from build123d import *

# Parameters (mm, degrees)
SKETCH1_R               = 1.995
BOSS_EXTRUDE1_DEPTH     = 38
SKETCH2_W               = 4.5
SKETCH2_H               = 0.920377874
CUT_EXTRUDE1_DEPTH      = 2.995
CUT_EXTRUDE1_DEPTH_BACK = 2.995
CHAMFER1_SIZE           = 0.2


with BuildPart() as part:
    # Sketch1 → Boss-Extrude1 (new body)
    with BuildSketch(Plane.XY):
        Circle(SKETCH1_R)
    extrude(amount=BOSS_EXTRUDE1_DEPTH)

    # Sketch2 → Cut-Extrude1 (cut, two sides)
    with BuildSketch(Plane(origin=(0, 0, 0), x_dir=(0, 0, -1), z_dir=(1, 0, 0))) as cut_extrude1_sk:
        with Locations((-3.75, 2.160188937)):
            Rectangle(SKETCH2_W, SKETCH2_H)
        with Locations((-3.75, -2.160188937)):
            Rectangle(SKETCH2_W, SKETCH2_H)
    extrude(amount=CUT_EXTRUDE1_DEPTH, mode=Mode.SUBTRACT)
    extrude(cut_extrude1_sk.sketch, amount=-CUT_EXTRUDE1_DEPTH_BACK, mode=Mode.SUBTRACT)

    # Chamfer1
    chamfer1_edges = [part.edges().sort_by_distance(p)[0] for p in [
        (-1.995, 0, 0),
        (-1.995, 0, 38),
    ]]
    chamfer(chamfer1_edges, length=CHAMFER1_SIZE)


solid = part.part
Verification items for the finished model (mm, model axes). A direction names the side the tool comes from. Coordinates: 2 decimals unless noted, no trailing zeros. Order: outer loops, then holes, each group sorted by start corner. A loop starts at its lowest first (then second) coordinate and runs counter-clockwise, first axis right, second up. Notation, with made-up numbers: (69, 63.5) -> (115, 63.5) arc R19 cw to (115, 79.5) -> close; hole circle Ø8 at (-33, 2). An arc over 180 degrees is marked (long way). Put each result on its own line as item: value. Start each with the question number.
1. Cross-section at A-A, the plane x = 0. Record the boundary of the cut face in (y, z) (3 decimals), then the cut area to 3 significant figures.
2. Cross-section at B-B, the plane z = 15. Record the boundary of the cut face in (x, y) (3 decimals), then the cut area to 3 significant figures.
3. Go/stop test with flat-tipped pins: pin 1 Ø1 at (x, z) = (1, 27) entering from -Y; pin 2 Ø1.5 at (x, z) = (-1.5, 9) entering from -Y; pin 3 Ø0.6 at (x, z) = (0, 3) entering from +Y. Record where each tip stops, or that it passes through.
4. Material ranges on L1, parallel to Y at x = 0.1, z = 17.5; L2, parallel to X at y = -1.05, z = 22; L3, parallel to Y at x = 1.4, z = 7, recorded low to high. Write a range as [from, to].
5. Mould release check, pull along Z, two halves, no side actions. Record for faces 1 (the cylindrical face through (-0.26, 1.98, 18.74)), 2 (the flat face through (0, 0, 38)), 3 (the flat face through (0, -1.7, 4)): released by +Z, released by -Z, zero draft, split by the parting line, or undercut.
6. Access from +Z, -Z, +X, -X, +Y, -Y to the whole of each face (thin tool, end or side, straight path). Record for faces 4 (the flat face through (0, 0, 0)), 5 (the flat face through (0, 1.7, 4)).
7. Cross-section at C-C, the plane z = 5.5. Record the boundary of the cut face in (x, y) (3 decimals), then the cut area to 3 significant figures.
Computed:
1. outline: (-1.995, 0.2) -> (-1.795, 0) -> (1.795, 0) -> (1.995, 0.2) -> (1.995, 1.5) -> (1.7, 1.5) -> (1.7, 6) -> (1.995, 6) -> (1.995, 37.8) -> (1.795, 38) -> (-1.795, 38) -> (-1.995, 37.8) -> (-1.995, 6) -> (-1.7, 6) -> (-1.7, 1.5) -> (-1.995, 1.5) -> close
1. area: 149 mm2
2. outline: circle Ø3.99 at (0, 0)
2. area: 12.5 mm2
3. pin 1: y = -1.93
3. pin 2: y = -1.85
3. pin 3: y = 1.7
4. L1: [-1.99, 1.99]
4. L2: [-1.7, 1.7]
4. L3: [-1.42, 1.42]
5. face 1: zero draft
5. face 2: released by +Z
5. face 3: undercut
6. face 4: -Z, +X, -X, +Y, -Y
6. face 5: +X, -X, +Y
7. outline: (-1.044, -1.7) -> (1.044, -1.7) arc R1.995 ccw to (1.044, 1.7) -> (-1.044, 1.7) arc R1.995 ccw to start
7. area: 11.7 mm2
